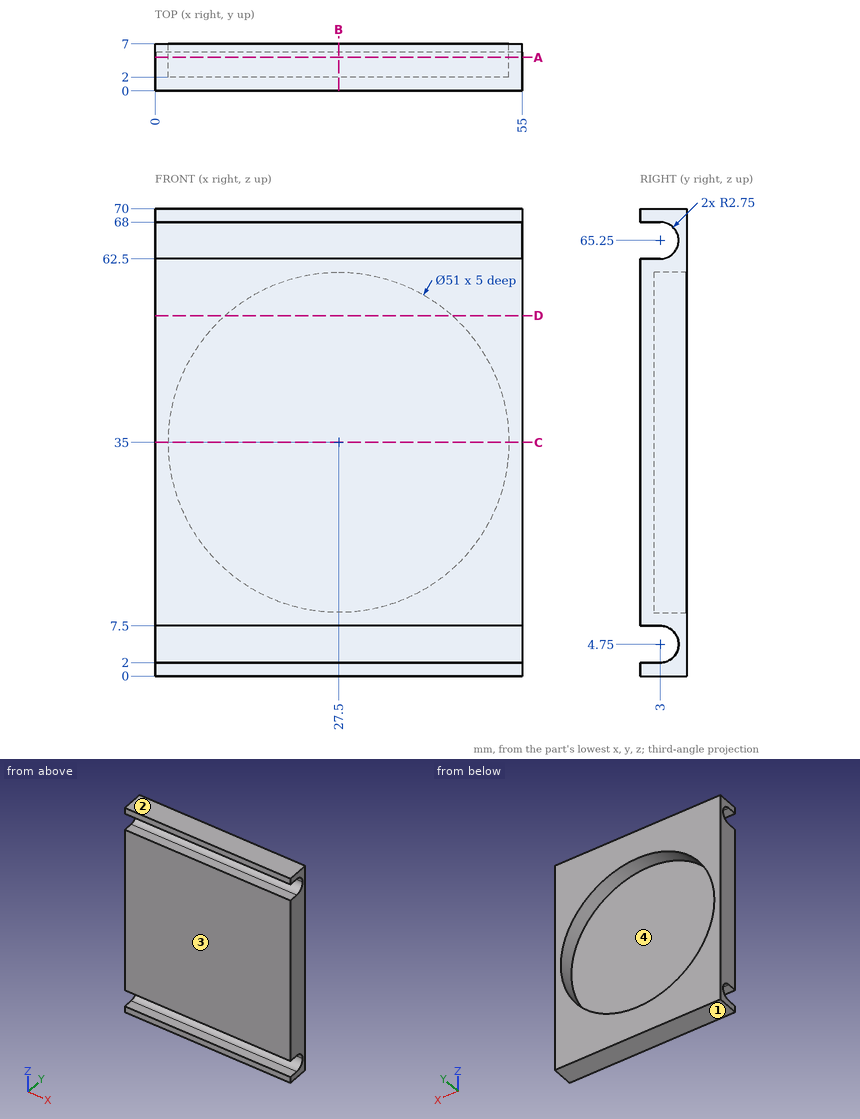
Answer from the drawing. Dimensions are ordinates in mm from the lowest x, y and z of the part. Coordinates: 2 decimals unless noted, no trailing zeros. Order: outer loops, then holes, each group sorted by start corner. A loop starts at its lowest first (then second) coordinate and runs counter-clockwise, first axis right, second up. Notation, with made-up numbers: (38.25, 4.25) -> (85.25, 4.25) arc R26 cw to (85.25, 37.25) -> close; hole circle Ø9 at (-32.5, 49). An arc over 180 degrees is marked (long way). Answer as a JSON object with one key per item and string values.
1) A cutting plane is placed at C-C, the plane z = 35. Determine the outline of the cut face in (x, y), plus the area to 3 significant figures.
Model answer:
{"outline": "(0, 0) -> (55, 0) -> (55, 7) -> (53, 7) -> (53, 2) -> (2, 2) -> (2, 7) -> (0, 7) -> close", "area": "130 mm²"}
2) This flat-tipped pin is pushed along its axis until it touches: pin 1 (6 mm diameter, centred on x = 24.5, z = 51, fed in from +Y). Where does it stop, or does it pass through?
Model answer:
{"pin 1": "stops at y = 2"}
3) A cutting plane is placed at A-A, the plane y = 5. Determine the outline of the cut face in (x, z), plus the area to 3 significant figures.
Model answer:
{"outline": "(0, 0) -> (55, 0) -> (55, 2.86) -> (0, 2.86) -> close; (0, 6.64) -> (55, 6.64) -> (55, 63.36) -> (0, 63.36) -> close; (0, 67.14) -> (55, 67.14) -> (55, 70) -> (0, 70) -> close; hole circle Ø51 at (27.5, 35)", "area": "1,390 mm²"}
4) A cutting plane is placed at D-D, the plane z = 54. Determine the outline of the cut face in (x, y), plus the area to 3 significant figures.
Model answer:
{"outline": "(0, 0) -> (55, 0) -> (55, 7) -> (44.51, 7) -> (44.51, 2) -> (10.49, 2) -> (10.49, 7) -> (0, 7) -> close", "area": "215 mm²"}
5) The mould has two halves that part along Z. Classify the marked faces 1, 2, 3 and 4: released by +Z, released by -Z, zero draft, split by the parting line, or undercut.
Model answer:
{"face 1": "released by -Z", "face 2": "released by +Z", "face 3": "zero draft", "face 4": "undercut"}
6) Consider line 1 along Z through (x, y) = (51.5, 1.25); line 2 along X through (y, z) = (4.95, 35); line 3 along Z through (x, y) = (40.5, 2.5). Determine where each line is inside the solid, lowest interval first. Write a range as from..to.
Model answer:
{"line 1": "z = 0..2, 7.5..62.5, 68..70", "line 2": "x = 0..2, 53..55", "line 3": "z = 0..2, 7.5..13.06, 56.94..62.5, 68..70"}
7) A cutting plane is placed at B-B, the plane x = 27.5. Determine the outline of the cut face in (y, z).
Model answer:
{"outline": "(0, 0) -> (7, 0) -> (7, 9.5) -> (2, 9.5) -> (2, 60.5) -> (7, 60.5) -> (7, 70) -> (0, 70) -> (0, 68) -> (3, 68) arc R2.75 cw to (3, 62.5) -> (0, 62.5) -> (0, 7.5) -> (3, 7.5) arc R2.75 cw to (3, 2) -> (0, 2) -> close"}
